Verification items for the finished model (mm, model axes). A direction names the side the tool comes from. Coordinates: 2 decimals unless noted, no trailing zeros. Loops run counter-clockwise (first coordinate to the right, second up) from the corner with the lowest first, then second, coordinate; pieces in that order, holes last. Notation, with made-up numbers: M 82.5,-34 L 104.5,-34 A19 ccw 104.5,-22 Z; hole C 6.25,74 d7. An arc over 180 degrees is marked long. Write item = value, one per line. Start each with the question number.
```python
from build123d import *

# Parameters (mm, degrees)
EXTRUDE_1_DEPTH     = 5
SKETCH_2_W          = 90
SKETCH_2_H          = 90
EXTRUDE_2_DEPTH     = 25
SKETCH_3_W          = 82.667839838
SKETCH_3_H          = 15.058257345
CUT_EXTRUDE_1_DEPTH = 90
SKETCH_4_W          = 82.085695662
SKETCH_4_H          = 16.995101666
CUT_EXTRUDE_2_DEPTH = 90
SKETCH_5_W          = 97.364780094
SKETCH_5_H          = 98.94366842
EXTRUDE_3_DEPTH     = 20
FILLET_1_R          = 10
SKETCH_6_W          = 90
SKETCH_6_H          = 90
EXTRUDE_4_DEPTH     = 30
CUT_EXTRUDE_3_DEPTH = 90
SKETCH_8_W          = 62.667839838
SKETCH_8_H          = 13.124346315
CUT_EXTRUDE_4_DEPTH = 10
CUT_EXTRUDE_5_DEPTH = 90
SKETCH_10_W         = 62.085695662
SKETCH_10_H         = 21.626220655
CUT_EXTRUDE_6_DEPTH = 10
SKETCH_11_W         = 62.667839838
SKETCH_11_H         = 13.124346315
CUT_EXTRUDE_7_DEPTH = 10
SKETCH_12_W         = 62.085695662
SKETCH_12_H         = 21.626220655
CUT_EXTRUDE_8_DEPTH = 10
EXTRUDE_5_DEPTH     = 20
SKETCH_14_R         = 36.481947273
EXTRUDE_6_DEPTH     = 10
FILLET_2_R          = 3


with BuildPart() as part:
    # 草图1 → 凸台-拉伸1 (new body)
    with BuildSketch(Plane(origin=(0, 0, 0), x_dir=(1, 0, 0), z_dir=(0, 1, 0))):
        Polygon((0, 70.903454713), (0, 0), (70.90345471, 0), (70.90345471, 50.896669322), (70.90345471, 63.546624398), (70.90345471, 70.903454713), (63.546624395, 70.903454713), (50.896669319, 70.903454713), align=None)
        Polygon((72.962659229, 92.969444623), (50.896669319, 70.903454713), (63.546624395, 70.903454713), (79.287636767, 86.644467085), align=None)
        Polygon((70.90345471, 70.903454713), (70.90345471, 63.546624398), (86.644467082, 79.28763677), (79.287636767, 86.644467085), (63.546624395, 70.903454713), align=None)
        Polygon((70.90345471, 63.546624398), (70.90345471, 50.896669322), (92.96944462, 72.962659232), (86.644467082, 79.28763677), align=None)
        with BuildLine():
            ThreePointArc((242.661241038, 250.018071355), (240.67172678, 254.833829646), (239.993214606, 260))
            Line((239.993214606, 260), (72.962659229, 92.969444623))
            Line((72.962659229, 92.969444623), (79.287636767, 86.644467085))
            Line((79.287636767, 86.644467085), (242.661241038, 250.018071355))
        make_face()
        with BuildLine():
            Line((92.96944462, 72.962659232), (260, 239.993214612))
            ThreePointArc((260, 239.993214606), (254.833829644, 240.67172678), (250.018071352, 242.66124104))
            Line((250.018071352, 242.66124104), (86.644467082, 79.28763677))
            Line((86.644467082, 79.28763677), (92.96944462, 72.962659232))
        make_face()
        with BuildLine():
            Line((260, 252.643169688), (260, 239.993214612))
            ThreePointArc((260, 239.993214606), (274.146933622, 245.853066378), (280.006785394, 260))
            ThreePointArc((280.006785394, 260), (260, 280.006785394), (239.993214606, 260))
            Line((239.993214606, 260), (252.643169682, 260))
            Line((252.643169682, 260), (260, 260))
            Line((260, 260), (260, 252.643169688))
        make_face()
        with BuildLine():
            Line((252.643169682, 260), (239.993214606, 260))
            ThreePointArc((239.993214606, 260), (240.67172678, 254.833829646), (242.661241038, 250.018071355))
            Line((242.661241038, 250.018071355), (252.643169682, 260))
        make_face()
        with BuildLine():
            ThreePointArc((250.018071352, 242.66124104), (254.833829644, 240.67172678), (260, 239.993214606))
            Line((260, 239.993214612), (260, 252.643169688))
            Line((260, 252.643169688), (250.018071352, 242.66124104))
        make_face()
    extrude_1 = extrude(amount=EXTRUDE_1_DEPTH)

    # 镜向1: 凸台-拉伸1 across plane
    add(extrude_1.mirror(Plane(origin=(0, 5, 0), x_dir=(0, 0, 1), z_dir=(1, 0, 0))))

    # 镜向3: part across plane


with BuildPart() as part_1:
    add(part.part)
    add(part.part.mirror(Plane(origin=(0, 5, 0), x_dir=(1, 0, 0), z_dir=(0, 0, -1))))

    # 草图2 → 凸台-拉伸2 (add)
    with BuildSketch(Plane.XZ):
        Rectangle(SKETCH_2_W, SKETCH_2_H)
    extrude(amount=EXTRUDE_2_DEPTH)

    # 草图3 → 切除-拉伸1 (cut)
    with BuildSketch(Plane.XY.offset(45)):
        with Locations((0, -12.246888496)):
            Rectangle(SKETCH_3_W, SKETCH_3_H)
    extrude(amount=-CUT_EXTRUDE_1_DEPTH, mode=Mode.SUBTRACT)

    # 草图4 → 切除-拉伸2 (cut)
    with BuildSketch(Plane(origin=(45, 0, 0), x_dir=(0, 0, -1), z_dir=(1, 0, 0))):
        with Locations((0, -12.272398252)):
            Rectangle(SKETCH_4_W, SKETCH_4_H)
    extrude(amount=-CUT_EXTRUDE_2_DEPTH, mode=Mode.SUBTRACT)

    # 草图5 → 凸台-拉伸3 (add)
    with BuildSketch(Plane(origin=(0, 5, 0), x_dir=(1, 0, 0), z_dir=(0, 1, 0))):
        Rectangle(SKETCH_5_W, SKETCH_5_H)
    extrude(amount=EXTRUDE_3_DEPTH)

    # 圆角1
    fillet_1_edges = [part_1.edges().sort_by_distance(p)[0] for p in [
        (48.682390047, 15, 49.47183421),
        (48.682390047, 15, -49.47183421),
        (-48.682390047, 15, -49.47183421),
        (-48.682390047, 15, 49.47183421),
        (48.682390047, 25, 0),
        (0, 25, -49.47183421),
        (-48.682390047, 25, 0),
        (0, 25, 49.47183421),
    ]]
    fillet(fillet_1_edges, radius=FILLET_1_R)

    # 草图6 → 凸台-拉伸4 (add)
    with BuildSketch(Plane.XZ.offset(25)):
        Rectangle(SKETCH_6_W, SKETCH_6_H)
    extrude(amount=EXTRUDE_4_DEPTH)

    # 草图7 → 切除-拉伸3 (cut)
    with BuildSketch(Plane.XY.offset(45)):
        Polygon((-41.333919919, -25.414932676), (41.333919919, -25.414932676), (41.333919919, -49.347564191), (31.333919919, -49.347564191), (31.333919919, -36.223217876), (-31.333919919, -36.223217876), (-31.333919919, -49.347564191), (-41.333919919, -49.347564191), align=None)
    extrude(amount=-CUT_EXTRUDE_3_DEPTH, mode=Mode.SUBTRACT)

    # 草图8 → 切除-拉伸4 (cut)
    with BuildSketch(Plane.XY.offset(45)):
        with Locations((0, -42.785391034)):
            Rectangle(SKETCH_8_W, SKETCH_8_H)
    extrude(amount=-CUT_EXTRUDE_4_DEPTH, mode=Mode.SUBTRACT)

    # 草图9 → 切除-拉伸5 (cut)
    with BuildSketch(Plane(origin=(45, 0, 0), x_dir=(0, 0, -1), z_dir=(1, 0, 0))):
        Polygon((-41.042847831, -26.273596919), (-41.042847831, -50.943507888), (-31.042847831, -50.943507888), (-31.042847831, -29.317287233), (31.042847831, -29.317287233), (31.042847831, -50.943507888), (41.042847831, -50.943507888), (41.042847831, -26.273596919), align=None)
    extrude(amount=-CUT_EXTRUDE_5_DEPTH, mode=Mode.SUBTRACT)

    # 草图10 → 切除-拉伸6 (cut)
    with BuildSketch(Plane(origin=(45, 0, 0), x_dir=(0, 0, -1), z_dir=(1, 0, 0))):
        with Locations((0, -40.130397561)):
            Rectangle(SKETCH_10_W, SKETCH_10_H)
    extrude(amount=-CUT_EXTRUDE_6_DEPTH, mode=Mode.SUBTRACT)

    # 草图11 → 切除-拉伸7 (cut)
    with BuildSketch(Plane(origin=(0, 0, -45), x_dir=(-1, 0, 0), z_dir=(0, 0, -1))):
        with Locations((0, -42.785391034)):
            Rectangle(SKETCH_11_W, SKETCH_11_H)
    extrude(amount=-CUT_EXTRUDE_7_DEPTH, mode=Mode.SUBTRACT)

    # 草图12 → 切除-拉伸8 (cut)
    with BuildSketch(Plane.ZY.offset(45)):
        with Locations((0, -40.130397561)):
            Rectangle(SKETCH_12_W, SKETCH_12_H)
    extrude(amount=-CUT_EXTRUDE_8_DEPTH, mode=Mode.SUBTRACT)

    # 草图13 → 凸台-拉伸5 (add)
    with BuildSketch(Plane.XY.offset(70.903454713)):
        Polygon((0, 0), (-10, 0), (-10, 5), (10, 5), (10, 0), align=None)
    extrude(amount=EXTRUDE_5_DEPTH)

    # 草图14 → 凸台-拉伸6 (add)
    with BuildSketch(Plane(origin=(0, 25, 0), x_dir=(1, 0, 0), z_dir=(0, 1, 0))):
        with Locations(Location((0, 0, 0), (0, 0, 270))):
            Circle(SKETCH_14_R)
    extrude(amount=EXTRUDE_6_DEPTH)

    # 圆角2
    fillet_2_edges = [part_1.edges().sort_by_distance(p)[0] for p in [
        (0, 35, -36.481947273),
    ]]
    fillet(fillet_2_edges, radius=FILLET_2_R)


solid = part_1.part
```
Q1. Gauge pin test, flat ends, axial feed: pin 1 (5 mm diameter, centred on y = -1, z = 98.5, fed in from +X); pin 2 (14.5 mm diameter, centred on y = -41, z = -15.5, fed in from +X); pin 3 (16.5 mm diameter, centred on x = 12.5, y = -33, fed in from -Z). Record the tip position at first contact, or that the pin passes through.
Q2. Mould release check, pull along Y, two halves, no side actions. Record for faces 6 (the face through (-35, 25, -12)), 7 (the face through (0, -20, 41.043)), 8 (the face through (-146.769, 2.465, -166.775)): +Y half, -Y half, draft (parallel to the pull), parting line (faces both ways), or undercut.
Q3. Sectioned sample at A-A on z = 0. Count the separate pieces of the cut face and the enclosed holes in it, plus the area to 3 significant figures.
Q4. Set-up check for faces 1 (the face through (0, -50, 41.043)), 2 (the face through (-1, -25.415, 1)), 3 (the face through (-146.769, 2.465, 166.775)), 4 (the face through (45, -25, 3)), 5 (the face through (-174.536, 2.465, 167.179)): record each of +Z, -Z, +X, -X, +Y, -Y from which the full face is reachable in a straight line by a thin tool's end or side.
Q5. Scan lines: L1, parallel to X at y = 12, z = -21; L2, parallel to X at y = 3, z = 155; L3, parallel to Y at x = 3.5, z = 87. Record each from-to range of solid material in increasing order. Write a range as [from, to].
Q6. Sectioned sample at C-C on z = 166.5. Record the cut outline in (x, y).
Q7. Sectioned sample at B-B on x = 158.5. Record the cut outline in (y, z), plus the area to 3 significant figures.
Solutions:
q1.pin_1 = 120.8
q1.pin_2 = 31.33
q1.pin_3 = -45
q2.face_6 = +Y half
q2.face_7 = undercut
q2.face_8 = draft
q3.separate_pieces = 3
q3.enclosed_holes = 0
q3.area = 5,400 mm²
q4.face_1 = +X, -X
q4.face_2 = +Z, -Z
q4.face_3 = +Z, +Y, -Y
q4.face_4 = +Z, -Z, +X, -Y
q4.face_5 = +Y, -Y
q5.L1 = [-48.68, 48.68]
q5.L2 = [-175.01, -162.36], [-147.64, -134.99], [134.99, 147.64], [162.36, 175.01]
q5.L3 = [0, 5]
q6.outline = M -186.51,0 L -173.86,0 L -173.86,5 L -186.51,5 Z; M -159.14,0 L -146.49,0 L -146.49,5 L -159.14,5 Z; M 146.49,0 L 159.14,0 L 159.14,5 L 146.49,5 Z; M 173.86,0 L 186.51,0 L 186.51,5 L 173.86,5 Z
q7.outline = M 0,-178.51 L 5,-178.51 L 5,-165.86 L 0,-165.86 Z; M 0,-151.14 L 5,-151.14 L 5,-138.49 L 0,-138.49 Z; M 0,138.49 L 5,138.49 L 5,151.14 L 0,151.14 Z; M 0,165.86 L 5,165.86 L 5,178.51 L 0,178.51 Z
q7.area = 253 mm²
